CAD build for the part. Positions are in the model's coordinates, mm. A direction names the side the tool comes from. Give positions to 0.01 mm unless a question says otherwise; leave off trailing zeros. Write each loop counter-clockwise with the first axis right and the second up, starting at its lowest first coordinate (ties: lowest second). Pieces come first, ordered by that corner, then holes. Notation, with made-up numbers: (88, 31) - (139, 31) arc R31 ccw to (139, 68) - close; hole circle Ø8 at (35.25, 2). An arc over 180 degrees is marked (long way). Answer as a JSON object with one key per item and string values.
from build123d import *

# Parameters (mm, degrees)
PAD_DEPTH           = 50
PAD001_DEPTH        = 50
CHAMFER_SIZE        = 5
SKETCH015_R         = 6
POCKET005_DEPTH     = 10
LINEARPATTERN_COUNT = 4
LINEARPATTERN_PITCH = 130
SKETCH016_R         = 7
POCKET_DEPTH        = 20


with BuildPart() as part:
    # Sketch → Pad (new body)
    with BuildSketch(Plane.XY):
        with BuildLine():
            Line((-379.627892, 300), (16.06014, 22.936257))
            ThreePointArc((28, 0), (24.836303, 12.928961), (16.06014, 22.936257))
            Line((34, 0), (28, 0))
            ThreePointArc((34, 0), (30.158368, 15.699453), (19.501599, 27.85117))
            Line((19.501599, 27.85117), (-376.186433, 304.914912))
            Line((-376.186433, 304.914912), (-379.627892, 300))
        make_face()
    extrude(amount=PAD_DEPTH)

    # Sketch001 → Pad001 (join)
    with BuildSketch(Plane.XY):
        Polygon((-94.605757, 107.75), (-103.174645, 113.75), (-1.740569, 113.75), (-1.740569, 107.75), align=None)
        Polygon((-113.171681, 120.75), (-121.740569, 126.75), (-1.740569, 126.75), (-1.740569, 120.75), align=None)
    extrude(amount=PAD001_DEPTH)

    # Chamfer
    chamfer_edges = [part.edges().sort_by_distance(p)[0] for p in [
        (-1.740569, 123.75, 50),
        (-1.740569, 110.75, 50),
        (-1.740569, 110.75, 0),
        (-1.740569, 123.75, 0),
    ]]
    chamfer(chamfer_edges, length=CHAMFER_SIZE)

    # Sketch015 → Pocket005 (cut)
    with BuildSketch(Plane(origin=(22.943057, 32.766082, 0), x_dir=(-0.819152, 0.573576, 0), z_dir=(0.573576, 0.819152, 0))):
        with Locations((454.477006, 25)):
            Circle(SKETCH015_R)
    pocket005 = extrude(amount=-POCKET005_DEPTH, mode=Mode.SUBTRACT)

    # LinearPattern: Pocket005 ×4
    with Locations(*[Vector(0.819152, -0.573576, 0) * (i * LINEARPATTERN_PITCH) for i in range(1, LINEARPATTERN_COUNT)]):
        add(pocket005, mode=Mode.SUBTRACT)

    # Sketch016 (on Face9 of LinearPattern) → Pocket (cut)
    with BuildSketch(Plane(origin=(0, 126.75, 0), x_dir=(-1, 0, 0), z_dir=(0, 1, 0))):
        with Locations((26.740569, 25)):
            Circle(SKETCH016_R)
    extrude(amount=-POCKET_DEPTH, mode=Mode.SUBTRACT)

    # Mirrored: part across XZ


with BuildPart() as part_1:
    add(part.part)
    add(part.part.mirror(Plane.XZ))


solid = part_1.part
Item 1: Mould opens along Z. For faces 4 (the cylindrical face through (-25.223, 123.792, 18.166)), 5 (the flat face through (-184.554, -163.408, 24.65)), 6 (the flat face through (-97, 112, 0)) say: +Z half, -Z half, draft (parallel to the pull), parting line (faces both ways), or undercut.
Entries:
{"face 4": "undercut", "face 5": "draft", "face 6": "-Z half"}
Item 2: Cut at A-A (x = -205.5). Give the cut face in (y, z), and give its area (3 significant figures).
Entries:
{"outline": "(-185.4, 0) - (-178.07, 0) - (-178.07, 50) - (-185.4, 50) - close; (178.07, 0) - (185.4, 0) - (185.4, 50) - (178.07, 50) - close", "area": "732 mm2"}
Item 3: Flat gauge pins, fed straight in: P1, Ø8, axis at y = 229, z = 42.5, coming from the +X side; P2, Ø2, axis at y = 119, z = 17, coming from the -X side; P3, Ø25, axis at x = -83.5, z = 15, coming from the +Y side. Where does each tip first touch, or does it go through?
Entries:
{"P1": "x = -262.06", "P2": "x = -122.56", "P3": "y = 126.75"}
Item 4: Probe line 1 (Y direction, x = -231, z = 35); line 2 (Y direction, x = -5, z = 33.5); line 3 (Y direction, x = -139.5, z = 33.5). List the from-to ranges inside material, lowest first. Write a range as from..to.
Entries:
{"line 1": "-203.25..-195.93, 195.93..203.25", "line 2": "-126.75..-120.75, -113.75..-107.75, -45.01..-37.68, 37.68..45.01, 107.75..113.75, 120.75..126.75", "line 3": "-139.19..-131.86, 131.86..139.19"}
Item 5: Cut at D-D (y = -175). Give the cut face in (x, z).
Entries:
{"outline": "(-201.11, 0) - (-190.65, 0) - (-190.65, 50) - (-201.11, 50) - close"}
Item 6: Cut at C-C (z = 25). State how many separate pieces and enclosed holes the cut face has, and give its area (3 significant figures).
Entries:
{"separate pieces": "5", "enclosed holes": "0", "area": "7,990 mm2"}
Item 7: Cut at B-B (x = -56). Give the cut face in (y, z), and give its area (3 significant figures).
Entries:
{"outline": "(-126.75, 0) - (-120.75, 0) - (-120.75, 50) - (-126.75, 50) - close; (-113.75, 0) - (-107.75, 0) - (-107.75, 50) - (-113.75, 50) - close; (-80.72, 0) - (-73.39, 0) - (-73.39, 50) - (-80.72, 50) - close; (73.39, 0) - (80.72, 0) - (80.72, 50) - (73.39, 50) - close; (107.75, 0) - (113.75, 0) - (113.75, 50) - (107.75, 50) - close; (120.75, 0) - (126.75, 0) - (126.75, 50) - (120.75, 50) - close", "area": "1,930 mm2"}
Item 8: Which spindle directions (+Z, -Z, +X, -X, +Y, -Y) get a long thin tool onto all of the face, cutting with end or side? Do faces 1 (the flat face through (-63, 126.75, 25)), 2 (the cylindrical face through (-25.223, -110.792, 18.166)), 3 (the flat face through (-53, -113.75, 25)). Say none if no direction does.
Entries:
{"face 1": "+Z, -Z, +X, +Y", "face 2": "-Y", "face 3": "+Z, -Z, +X"}
